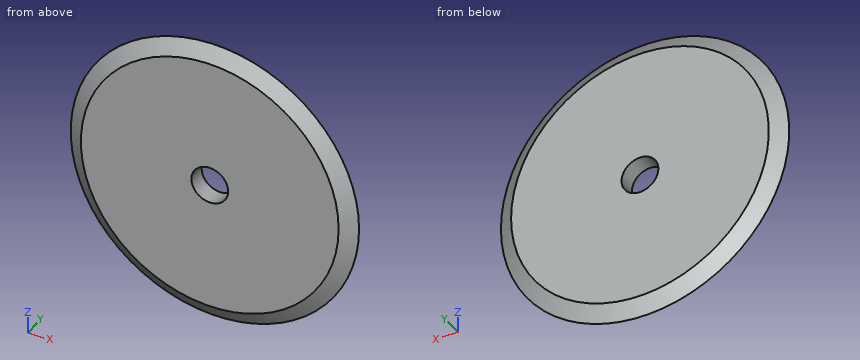
from build123d import *

# Parameters (mm, degrees)
F0_R     = 25.4
F0_R_2   = 3.175
F1_DEPTH = 3.048
F2_SIZE2 = 1.8330871047
F2_SIZE  = 3.175


# Not quite as in the source:
# - a fillet or chamfer that OpenCascade refuses, or shapes differently, is made with other operations: its cross-section is extruded or revolved along the edge and cut away or added


with BuildPart() as f1:
    # F0 (on Front) → F1 (new body)
    with BuildSketch(Plane.XZ):
        Circle(F0_R)
        Circle(F0_R_2, mode=Mode.SUBTRACT)
    extrude(amount=F1_DEPTH)

    # F2
    f2_edges = [f1.edges().sort_by_distance(p)[0] for p in [
        (-25.4, -3.048, 0),
    ]]
    f2_side = f1.faces().sort_by_distance((-24.68158, -3.048, 0))[0]
    chamfer(f2_edges, length=F2_SIZE, length2=F2_SIZE2, reference=f2_side)

    # F3: chamfer of 3.175 x 1.8330871047 on 1 edges, made by hand

    # F3_s1 → F3_t2 (revolve, cut)
    with BuildSketch(Plane.XY):
        Polygon((25.4, -1.8330871047), (22.225, 0), (25.4, 0), align=None)
    revolve(axis=Axis((0, 0, 0), (0, -1, 0)), mode=Mode.SUBTRACT)


solid = f1.part
Can you work these out from the model? Positions are in its coordinate system, mm. Give positions to 0.01 mm unless a question says otherwise; leave off trailing zeros. Write each loop counter-clockwise with the first axis right and the second up, starting at its lowest first coordinate (ties: lowest second). Pieces come first, ordered by that corner, then holes. Notation, with made-up numbers: M 76.5,11.25 L 82.5,11.25 A27 cw 82.5,41.25 Z; hole C 46,84.25 d1. An arc over 180 degrees is marked long. Answer in a Markdown table with one row per item. Add a question column.
Item 1: Imagine slicing it at B-B, the plane x = 0. Write out the boundary of the cut face in (y, z) (3 decimals), plus the area to 3 significant figures.
Item 2: Imagine slicing it at C-C, the plane y = -1.05. Write out the boundary of the cut face in (x, z) (3 decimals), plus the area to 3 significant figures.
Item 3: Imagine slicing it at A-A, the plane z = 0. Write out the boundary of the cut face in (x, y) (3 decimals), plus the area to 3 significant figures.
Item 4: Please list where these lines run through material, in increasing order: L1, parallel to X at y = -2.15, z = -2.5; L2, parallel to Z at x = -1.5, y = -2.5; L3, parallel to Z at x = -7.5, y = -0.7.
Evaluation:
| question | item | result |
|---|---|---|
| 1 | outline | M -3.048,-22.225 L -1.524,-24.865 L 0,-22.225 L 0,-3.175 L -3.048,-3.175 Z; M -3.048,3.175 L 0,3.175 L 0,22.225 L -1.524,24.865 L -3.048,22.225 Z |
| 1 | area | 124 mm² |
| 2 | outline | C 0,0 d48.087; hole C 0,0 d6.35 |
| 2 | area | 1,780 mm² |
| 3 | outline | M -24.865,-1.524 L -22.225,-3.048 L -3.175,-3.048 L -3.175,0 L -22.225,0 Z; M 3.175,-3.048 L 22.225,-3.048 L 24.865,-1.524 L 22.225,0 L 3.175,0 Z |
| 3 | area | 124 mm² |
| 4 | L1 | x = -23.65 to -1.96, 1.96 to 23.65 |
| 4 | L2 | z = -23.13 to -2.8, 2.8 to 23.13 |
| 4 | L3 | z = -22.21 to 22.21 |
